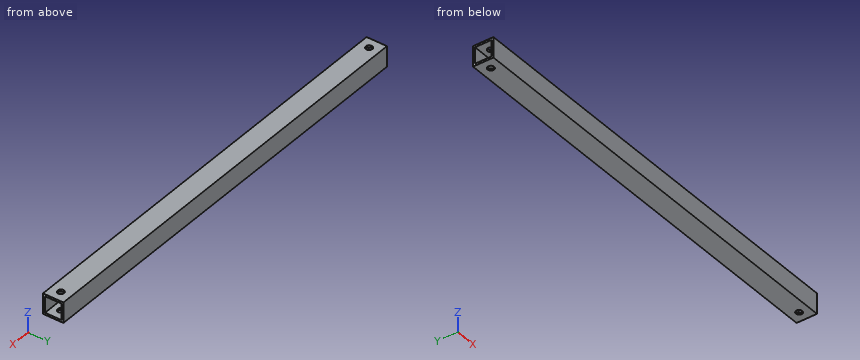
```python
from build123d import *

# Parameters (mm, degrees)
SKETCH_1_W          = 210.89955229
SKETCH_1_H          = 10
SKETCH_1_R          = 1.6
SKETCH_1_R_2        = 1.559795767
EXTRUDE_1_DEPTH     = 10
SKETCH_2_W          = 8
SKETCH_2_H          = 8
CUT_EXTRUDE_1_DEPTH = 507.140910376


with BuildPart() as part:
    # ｽｹｯﾁ1 → ﾎﾞｽ - 押し出し1 (new body)
    with BuildSketch(Plane.XY):
        with Locations((-466.84495805, 455)):
            Rectangle(SKETCH_1_W, SKETCH_1_H)
        with Locations((-567.294734195, 455)):
            Circle(SKETCH_1_R, mode=Mode.SUBTRACT)
        with Locations((-366.395181905, 454.995481815)):
            Circle(SKETCH_1_R_2, mode=Mode.SUBTRACT)
    extrude(amount=EXTRUDE_1_DEPTH)

    # ｽｹｯﾁ2 → ｶｯﾄ - 押し出し1 (cut, through all)
    with BuildSketch(Plane.ZY.offset(572.294734195)):
        with Locations((5, 455)):
            Rectangle(SKETCH_2_W, SKETCH_2_H)
    extrude(amount=-CUT_EXTRUDE_1_DEPTH, mode=Mode.SUBTRACT)


solid = part.part
```
Read the model definition and answer for the solid it produces. Units are mm, in the model's axes. Coordinates: 2 decimals unless noted, no trailing zeros. Write each loop counter-clockwise with the first axis right and the second up, starting at its lowest first coordinate (ties: lowest second). Pieces come first, ordered by that corner, then holes. Notation, with made-up numbers: (74.5, 84) -> (89.5, 84) arc R19 cw to (89.5, 117) -> close; hole circle Ø4 at (89.25, -37). An arc over 180 degrees is marked (long way). Answer as a JSON object with one key per item and string values.
Q1. Consider line 1 (X direction, y = 455, z = 0.65); line 2 (Y direction, x = -388, z = 4.25); line 3 (Z direction, x = -496, y = 454.75). Determine where each line is inside the solid, lowest interval first. Write a range as [from, to].
The answers:
{"line 1": "x = [-572.29, -568.89], [-565.69, -367.95], [-364.84, -361.4]", "line 2": "y = [450, 451], [459, 460]", "line 3": "z = [0, 1], [9, 10]"}
Q2. A flat-ended cylindrical pin translates along its axis: pin 1 Ø5 at (y, z) = (458, 5.5) entering from +X. Find the tip coordinate at first contact, or state that the pin passes through.
The answers:
{"pin 1": "stops at x = -361.4"}
Q3. The part is cut by section A-A on z = 4.75. Give the vertices of the cut face in (x, y), then the cut area to 3 significant figures.
The answers:
{"outline": "(-572.29, 450) -> (-361.4, 450) -> (-361.4, 451) -> (-572.29, 451) -> close; (-572.29, 459) -> (-361.4, 459) -> (-361.4, 460) -> (-572.29, 460) -> close", "area": "422 mm2"}
Q4. The part is cut by section B-B on x = -472. Give the vertices of the cut face in (y, z).
The answers:
{"outline": "(450, 0) -> (460, 0) -> (460, 10) -> (450, 10) -> close; hole (451, 1) -> (459, 1) -> (459, 9) -> (451, 9) -> close"}
